The model under review builds one solid part; all positions refer to its coordinate system, in mm. Round coordinates to 2 decimals unless told otherwise and drop trailing zeros. Write each loop counter-clockwise with the first axis right and the second up, starting at its lowest first coordinate (ties: lowest second). Pieces come first, ordered by that corner, then holes. Notation, with made-up numbers: (-12.75, 51.25) -> (-3.75, 51.25) arc R22 ccw to (-3.75, 66.25) -> close; hole circle Ø2 at (83.5, -23). An arc over 180 degrees is marked (long way). Answer in a Markdown table with one row per item. Add a question column.
```python
from build123d import *

# Parameters (mm, degrees)
EXTRUDE_1_DEPTH = 1
EXTRUDE_2_DEPTH = 1


with BuildPart() as part:
    # 草图2 → 凸台-拉伸1 (new body)
    with BuildSketch(Plane(origin=(0, 0, 0), x_dir=(1, 0, 0), z_dir=(0, 1, 0))):
        with BuildLine():
            Line((-37.75, -5.187524662), (-37.427791342, -12.336938121))
            Line((-37.427791342, -12.336938121), (-30.410766277, -53.09868086))
            ThreePointArc((-30.410766277, -53.09868086), (0, -28.114102247), (30.410766277, -53.09868086))
            Line((30.410766277, -53.09868086), (36.657098941, -16.813873157))
            Line((36.657098941, -16.813873157), (37.001393596, -14.813873158))
            Line((37.001393596, -14.813873158), (-21.5, -14.813873158))
            Line((-21.5, -14.813873158), (-21.5, -1.937524662))
            Line((-21.5, -1.937524662), (-37.75, -1.937524662))
            Line((-37.75, -1.937524662), (-37.75, -5.187524662))
        make_face()
    extrude(amount=EXTRUDE_1_DEPTH)

    # 草图3 → 凸台-拉伸2 (add)
    # profile 1 of 2: a face of its own
    with BuildSketch(Plane(origin=(0, 0, 0), x_dir=(1, 0, 0), z_dir=(0, 1, 0))):
        with BuildLine():
            Line((-0.856008306, -26.09621982), (-1.623205137, -26.09621982))
            Line((-1.623205137, -26.09621982), (-1.623205137, -24.137821353))
            add(Edge.make_bspline(
                [(-1.623205137, -24.137821353), (-1.655268125, -24.143514077), (-1.721316296, -24.155240806), (-1.824283839, -24.164783502), (-1.933346323, -24.17076586), (-2.008053511, -24.170657837), (-2.046485638, -24.170602266)],
                knots=[0, 0, 0, 0, 0.918585764, 1.892241272, 2.915691322, 4, 4, 4, 4], degree=3))
            add(Edge.make_bspline(
                [(-2.046485638, -24.170602266), (-2.104785366, -24.170571941), (-2.220025321, -24.170511997), (-2.390487029, -24.154509017), (-2.556692953, -24.12850453), (-2.718324735, -24.089526065), (-2.87582336, -24.039158247), (-3.029314168, -23.977977332), (-3.17798521, -23.903769977), (-3.321131503, -23.818737452), (-3.455836859, -23.720606314), (-3.573248856, -23.603221137), (-3.675029776, -23.4704659), (-3.7579419, -23.320396932), (-3.825592093, -23.154649423), (-3.874729538, -22.972446384), (-3.908442208, -22.774352183), (-3.916101546, -22.636664835), (-3.920068751, -22.565348758)],
                knots=[0, 0, 0, 0, 1.003522523, 1.98364375, 2.944869411, 3.898614004, 4.843729631, 5.790462383, 6.741287792, 7.702146141, 8.655643954, 9.602935836, 10.551034771, 11.527201242, 12.5464735, 13.626777097, 14.770773406, 16, 16, 16, 16], degree=3))
            add(Edge.make_bspline(
                [(-3.920068751, -22.565348758), (-3.917621314, -22.509206105), (-3.912856522, -22.399904758), (-3.888966748, -22.241365875), (-3.851887205, -22.092719231), (-3.802758946, -21.953287322), (-3.736987826, -21.824826369), (-3.660822021, -21.704776101), (-3.569736975, -21.595056691), (-3.499181783, -21.53152241), (-3.46371946, -21.499588924)],
                knots=[0, 0, 0, 0, 1.126595518, 2.193312949, 3.209115705, 4.196248007, 5.151139266, 6.097382339, 7.043709754, 8, 8, 8, 8], degree=3))
            add(Edge.make_bspline(
                [(-3.46371946, -21.499588924), (-3.423819299, -21.467392586), (-3.342763644, -21.401986955), (-3.204758648, -21.32105817), (-3.053205789, -21.252406965), (-2.887562725, -21.19534799), (-2.707183639, -21.152151647), (-2.5123955, -21.123211501), (-2.303575344, -21.103250861), (-2.159600384, -21.101683502), (-2.085223363, -21.100873809)],
                knots=[0, 0, 0, 0, 0.838628006, 1.70364077, 2.610636308, 3.559859354, 4.568055018, 5.643200099, 6.782484425, 8, 8, 8, 8], degree=3))
            add(Edge.make_bspline(
                [(-2.085223363, -21.100873809), (-2.022547246, -21.101999243), (-1.900326605, -21.10419388), (-1.722031706, -21.10963235), (-1.553493577, -21.11799829), (-1.394779498, -21.129605553), (-1.245704987, -21.14233845), (-1.106447222, -21.158428618), (-0.977269579, -21.177092329), (-0.894709866, -21.191984217), (-0.855064406, -21.199135354)],
                knots=[0, 0, 0, 0, 1.217605855, 2.374374404, 3.464660226, 4.494999595, 5.465333604, 6.370582827, 7.217548217, 8, 8, 8, 8], degree=3))
            Line((-0.855064406, -21.199135354), (-0.856008306, -26.09621982))
        make_face()
        with BuildLine():
            add(Edge.make_bspline(
                [(-1.623205137, -21.739832201), (-1.65274721, -21.733999838), (-1.719633086, -21.720794849), (-1.833986924, -21.708704947), (-1.973601931, -21.699443395), (-2.075441396, -21.696669118), (-2.130574845, -21.695167191)],
                knots=[0, 0, 0, 0, 0.708180311, 1.603383121, 2.702528978, 4, 4, 4, 4], degree=3))
            add(Edge.make_bspline(
                [(-2.130574845, -21.695167191), (-2.168073561, -21.695952692), (-2.24132842, -21.697487191), (-2.348460101, -21.707705221), (-2.449759776, -21.725860501), (-2.54572877, -21.750031884), (-2.635478405, -21.782226009), (-2.71969003, -21.821293247), (-2.797963445, -21.867371353), (-2.870093205, -21.92060581), (-2.935949572, -21.979929245), (-2.993080877, -22.047665882), (-3.041017981, -22.122592696), (-3.081384443, -22.203868683), (-3.112473184, -22.292435582), (-3.13480904, -22.388111375), (-3.14923784, -22.490598656), (-3.151639324, -22.56120559), (-3.152872842, -22.597472724)],
                knots=[0, 0, 0, 0, 1.164286524, 2.274468469, 3.33712435, 4.356941393, 5.343590938, 6.292901648, 7.23538906, 8.158502959, 9.072142365, 9.981112688, 10.900594105, 11.827687296, 12.792632354, 13.80775062, 14.873954761, 16, 16, 16, 16], degree=3))
            add(Edge.make_bspline(
                [(-3.152872842, -22.597472724), (-3.151613433, -22.636249876), (-3.149167963, -22.711545774), (-3.13519411, -22.82079109), (-3.111174009, -22.922850983), (-3.079419521, -23.018294919), (-3.038824966, -23.107069292), (-2.988156623, -23.188218343), (-2.928144539, -23.262075146), (-2.860007553, -23.329662929), (-2.783057089, -23.388781734), (-2.699594044, -23.441477416), (-2.608012254, -23.4847832), (-2.509562282, -23.520465241), (-2.404100063, -23.54918737), (-2.291122917, -23.56840422), (-2.171164858, -23.580930403), (-2.088720416, -23.582872542), (-2.046485638, -23.583867464)],
                knots=[0, 0, 0, 0, 1.10647952, 2.148516939, 3.135813804, 4.093347323, 5.013956832, 5.913991464, 6.814877829, 7.723438285, 8.645449828, 9.577866136, 10.534345172, 11.529217628, 12.562346088, 13.648092354, 14.795160789, 16, 16, 16, 16], degree=3))
            add(Edge.make_bspline(
                [(-2.046485638, -23.583867464), (-2.00521482, -23.584412899), (-1.926388911, -23.585454662), (-1.814442024, -23.578443617), (-1.714043734, -23.567445346), (-1.652392814, -23.552941286), (-1.623205137, -23.546074562)],
                knots=[0, 0, 0, 0, 1.161518353, 2.218461969, 3.156558288, 4, 4, 4, 4], degree=3))
            Line((-1.623205137, -23.546074562), (-1.623205137, -21.739832201))
        make_face(mode=Mode.SUBTRACT)
    # profile 2 of 2: a face of its own
    with BuildSketch(Plane(origin=(0, 0, 0), x_dir=(1, 0, 0), z_dir=(0, 1, 0))):
        with BuildLine():
            Line((0.130386434, -21.131914551), (0.897583266, -21.131914551))
            Line((0.897583266, -21.131914551), (0.897583266, -24.155636425))
            add(Edge.make_bspline(
                [(0.897583266, -24.155636425), (0.89929321, -24.215445763), (0.902592367, -24.33084157), (0.915368258, -24.497724176), (0.936829282, -24.652102877), (0.966769663, -24.79430293), (1.005239493, -24.924351911), (1.052260261, -25.041802473), (1.107369405, -25.147128319), (1.170551424, -25.240289062), (1.242373791, -25.321087274), (1.319851887, -25.391822873), (1.404784791, -25.450371121), (1.495300915, -25.499626189), (1.593035117, -25.536183316), (1.69708966, -25.5615439), (1.807291946, -25.577012589), (1.882979468, -25.57854654), (1.921769062, -25.579332685)],
                knots=[0, 0, 0, 0, 1.442558911, 2.783265207, 4.033293762, 5.19797452, 6.283894868, 7.299176403, 8.243481286, 9.144954945, 10.005756174, 10.844503658, 11.66816234, 12.486940923, 13.323278702, 14.176003432, 15.065208066, 16, 16, 16, 16], degree=3))
            add(Edge.make_bspline(
                [(1.921769062, -25.579332685), (1.957725333, -25.578915325), (2.028096046, -25.578098501), (2.130909973, -25.562628358), (2.228129718, -25.535898617), (2.320368479, -25.498795392), (2.40757394, -25.451723675), (2.488940384, -25.393059054), (2.564744704, -25.323401018), (2.635860422, -25.243242907), (2.699760366, -25.150387865), (2.755013907, -25.045271413), (2.802850288, -24.927654795), (2.840414423, -24.797263515), (2.872028446, -24.654713055), (2.894014576, -24.499623904), (2.908368244, -24.332115662), (2.910724859, -24.216299952), (2.911943092, -24.156429928)],
                knots=[0, 0, 0, 0, 0.880869997, 1.723967724, 2.54076827, 3.348096003, 4.15667844, 4.964596865, 5.80091263, 6.676282017, 7.586647838, 8.557371955, 9.582678263, 10.694376867, 11.880403812, 13.160330013, 14.532054847, 16, 16, 16, 16], degree=3))
            Line((2.911943092, -24.156429928), (2.911943092, -21.131914551))
            Line((2.911943092, -21.131914551), (3.679139924, -21.131914551))
            Line((3.679139924, -21.131914551), (3.679139924, -24.109921407))
            add(Edge.make_bspline(
                [(3.679139924, -24.109921407), (3.677188401, -24.198867937), (3.673417448, -24.370740501), (3.648553918, -24.618287645), (3.610391814, -24.846397955), (3.557827499, -25.055163342), (3.491261126, -25.245040827), (3.410030292, -25.415512075), (3.31448028, -25.566466666), (3.203498097, -25.697108223), (3.080569907, -25.809550333), (2.94882349, -25.908176054), (2.805519828, -25.989407969), (2.653202823, -26.056947418), (2.49058693, -26.108131021), (2.318208544, -26.142255886), (2.1365007, -26.164139495), (2.011908047, -26.164790111), (1.948224093, -26.165122665)],
                knots=[0, 0, 0, 0, 1.389947096, 2.68581329, 3.884176986, 5.001519278, 6.046082896, 7.023506491, 7.946473535, 8.830015835, 9.69383004, 10.545329235, 11.396344648, 12.262399475, 13.145009074, 14.054291982, 15.00547603, 16, 16, 16, 16], degree=3))
            add(Edge.make_bspline(
                [(1.948224093, -26.165122665), (1.881721214, -26.164339998), (1.751827834, -26.162811293), (1.561981249, -26.141967577), (1.382440978, -26.104865244), (1.212643091, -26.053613752), (1.053287044, -25.984492529), (0.903741738, -25.900795559), (0.764964905, -25.800213917), (0.635145258, -25.685884953), (0.518115943, -25.552843022), (0.4164162, -25.399939828), (0.330633136, -25.227687461), (0.260185761, -25.036841598), (0.204398311, -24.827427738), (0.164915765, -24.598798774), (0.137702567, -24.351381444), (0.133499992, -24.179812722), (0.131330334, -24.091237172)],
                knots=[0, 0, 0, 0, 1.013962662, 1.980471211, 2.907472823, 3.806985122, 4.680561309, 5.551651082, 6.415505808, 7.289926821, 8.185106327, 9.109702809, 10.082849364, 11.113391155, 12.207519227, 13.383461846, 14.649163417, 16, 16, 16, 16], degree=3))
            Line((0.131330334, -24.091237172), (0.130386434, -21.131914551))
        make_face()
    extrude(amount=-EXTRUDE_2_DEPTH)


solid = part.part
```
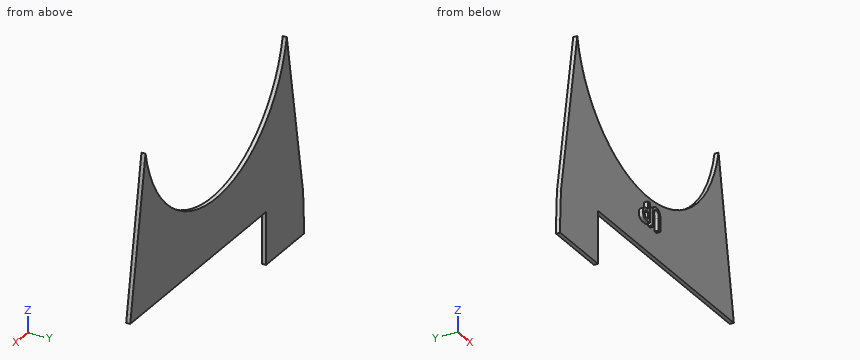
1. Add section C-C on z = 33. Write out the cut boundary in (x, y), plus the area to 3 significant figures.
2. Add section D-D on x = -24. Write out the cut boundary in (y, z).
3. Add section A-A on z = 41.5. Write out the cut boundary in (x, y).
4. For L1, parallel to X at y = -0.5, z = 23; L2, parallel to X at y = 0.1, z = 5; L3, parallel to X at y = 0.8, z = 44, list the stretches that pass through material, from the lowest coordinate up.
5. Insertion check: pin 1 Ø1.1 at (y, z) = (-0.5, 25) entering from -X; pin 2 Ø1 at (x, y) = (13, 0.5) entering from +Z; pin 3 Ø0.5 at (y, z) = (-0.5, 22.5) entering from -X; pin 4 Ø12 at (x, z) = (4, 37.5) entering from +Y. Each pin has a flat end and moves straight along its axis. Give the tip position at first contact, or say it passes through.
6. Add section B-B on y = 0.55. Write out the cut boundary in (x, z), plus the area to 3 significant figures.
Filled in:
| question | item | result |
|---|---|---|
| 1 | outline | (-33.87, 0) -> (-16.7, 0) -> (-16.7, 1) -> (-33.87, 1) -> close; (16.7, 0) -> (33.87, 0) -> (33.87, 1) -> (16.7, 1) -> close |
| 1 | area | 34.3 mm² |
| 2 | outline | (0, 1.94) -> (1, 1.94) -> (1, 39.49) -> (0, 39.49) -> close |
| 3 | outline | (-32.41, 0) -> (-25.51, 0) -> (-25.51, 1) -> (-32.41, 1) -> close; (25.51, 0) -> (32.41, 0) -> (32.41, 1) -> (25.51, 1) -> close |
| 4 | L1 | -3.87 to -3.08, -1.62 to -0.86, 0.13 to 0.9, 2.91 to 3.68 |
| 4 | L2 | -37.75 to -21.5 |
| 4 | L3 | -31.98 to -27.07, 27.07 to 31.98 |
| 5 | pin 1 | x = -35.29 |
| 5 | pin 2 | z = 31.21 |
| 5 | pin 3 | x = -3.92 |
| 5 | pin 4 | through |
| 6 | outline | (-37.75, 1.94) -> (-21.5, 1.94) -> (-21.5, 14.81) -> (37, 14.81) -> (30.41, 53.1) arc R31 cw to (-30.41, 53.1) -> (-37.43, 12.34) -> (-37.75, 5.19) -> close |
| 6 | area | 1,650 mm² |
